Build history of the part. All positions in model axes, mm. A direction names the side the tool comes from. Round coordinates to 2 decimals unless told otherwise and drop trailing zeros. Loops run counter-clockwise (first coordinate to the right, second up) from the corner with the lowest first, then second, coordinate; pieces in that order, holes last. Notation, with made-up numbers: (52, 32.5) -> (92, 32.5) arc R7 cw to (92, 38.5) -> close; hole circle Ø1 at (-10, -19). An arc over 180 degrees is marked (long way). Put each result on its own line as item: value. Start each with the question number.
Item 1: Pull direction Z, two halves, no side cores. Call faces 3 (the flat face through (3.042, 9.042, 5.172)), 4 (the flat face through (0.1, 23, -21.2)): +Z half, -Z half, draft (parallel to the pull), parting line (faces both ways), or undercut.
Item 2: Drill centre lines: probe 1 along Z at (x, y) = (0, 3.35); probe 2 along X at (y, z) = (7.75, -15); probe 3 along Z at (x, y) = (14.5, 7). Where is each one in solid material? Low to high. Write a range as [from, to].
Item 3: Tool access for faces 1 (the flat face through (1.5, 12, -6.3)), 2 (the flat face through (-3.898, 6.084, 13.613)): list every direction of +Z, -Z, +X, -X, +Y, -Y with a clear straight run to the whole face (end or side of a thin tool).
Item 4: Cut at A-A, the plane y = 8. Count the separate pieces of the cut face and the enclosed holes in it, plus the area to 3 significant figures.
Item 5: Cut at C-C, the plane y = 19.5. List the corners of the cut face in (x, z).
Item 6: Flat gauge pins, fed straight in: pin 1 Ø10 at (x, y) = (15, 18) entering from +Z; pin 2 Ø13 at (x, y) = (-12.5, 5) entering from -Z; pin 3 Ø9.5 at (x, z) = (-2, 0.5) entering from +Y. Where does each tip first touch, or does it go through?
Autodesk Inventor part; units mm, degrees
ref_plane "YZ Plane" through (0, 0, 0) normal (1, 0, 0) x (0, 1, 0)
ref_plane "XZ Plane" through (0, 0, 0) normal (0, 1, 0) x (-1, 0, 0)
ref_plane "XY Plane" through (0, 0, 0) normal (0, 0, 1) x (1, 0, 0)
sketch "草圖1" plane through (0, 0, 0) normal (0, 1, 0) x (-1, 0, 0)
  circle A0 centre (0, 0) radius 26
  dimension "d0" = 52
extrude "擠出1" add sketch "草圖1" along normal blind 23
fillet "圓角1" radius 2 2 edges at (26, 23, 0) (26, 0, 0)
sketch "草圖2" plane through (0, 23, 0) normal (0, 1, 0) x (1, 0, 0)
  circle A0 centre (0, 0) radius 21
  dimension "d4" = 42
extrude "擠出2" cut sketch "草圖2" against normal blind 11
sketch "草圖3" plane through (0, 12, 0) normal (0, 1, 0) x (1, 0, 0)
  circle A0 centre (0, 0) radius 8
  line L0 (-6, 3.4641) -> (0, 6.9282)
  line L1 (0, 6.9282) -> (6, 3.4641)
  line L2 (6, 3.4641) -> (6, -3.4641)
  line L3 (6, -3.4641) -> (0, -6.9282)
  line L4 (0, -6.9282) -> (-6, -3.4641)
  line L5 (-6, -3.4641) -> (-6, 3.4641)
  dimension "d7" = 12
  dimension "d8" = 16
extrude "擠出3" cut sketch "草圖3" against normal blind 6 contours L0 L1 L2 L3 L4 L5
sketch "草圖4" plane through (0, 12, 0) normal (0, 1, 0) x (1, 0, 0)
  circle A0 centre (0, 0) radius 21
  circle A1 centre (0, 0) radius 8
  line L0 (0, 0) -> (-21, 0)
  line L1 (0, 0) -> (-16.9894, 12.3435)
  circle A2 centre (0, 0) radius 21
  line L2 (-21, 0.5) -> (-1.5388, 0.5)
  line L3 (-1.5388, 0.5) -> (-17.2832, 11.939)
  circle A3 centre (0, 0) radius 20.5
  point P0 (-16.8738, 11.6415)
  point P1 (-20.4939, 0.5)
  point P2 (-7.9844, 0.5)
  point P3 (-6.7534, 4.2886)
  dimension "d11" = 36
  dimension "d12" = 0.5
  dimension "d13" = 0.5
extrude "擠出4" cut sketch "草圖4" against normal through all contours L3 A1 L2 A3
pattern_circular "環形陣列1" count 10 over 360 about axis through (0, -10, 0) along (0, 1, 0) of "擠出4"
sketch "草圖5" plane through (0, 6, 0) normal (0, 1, 0) x (1, 0, 0)
  circle A0 centre (0, 0) radius 2
  dimension "d19" = 4
extrude "擠出5" cut sketch "草圖5" against normal through all
sketch "草圖6" plane through (0, 23, 0) normal (0, 1, 0) x (1, 0, 0)
  circle A0 centre (0, 0) radius 26
  line L0 (48.5339, -26) -> (-4.5845, -26)
  line L1 (-4.5845, -26) -> (-136.2974, 21.9396)
  line L2 (0, 0) -> (-8.8925, -24.432)
  line L3 (0, 36.4) -> (0, -36.4)
  line L4 (4.5845, -26) -> (40.2795, -13.0081)
  dimension "d22" = 20
  dimension "d23" = 20
properties part number "wheel"
Reply:
1. face 3: undercut
1. face 4: draft
2. probe 1: z = [-26, -20.5], [-8, -2], [2, 8], [20.5, 26]
2. probe 2: x = [-21.24, -13.97], [-5.4, -4.35], [4.35, 5.4], [13.97, 21.24]
2. probe 3: z = [-21.58, -14.49], [-11.15, -9.92], [-0.5, 0.5], [9.92, 11.15], [14.49, 21.58]
3. face 1: +Y
3. face 2: +Y, -Y
4. separate pieces: 1
4. enclosed holes: 11
4. area: 1,000 mm^2
5. outline: circle Ø52 at (0, 0); hole circle Ø42 at (0, 0)
6. pin 1: stops at z = 24
6. pin 2: stops at z = -25.3
6. pin 3: stops at y = 12
